from build123d import *

# Parameters (mm, degrees)
CROQUIS1_R              = 60
SALIENTE_EXTRUIR1_DEPTH = 2
CROQUIS2_R              = 60
CROQUIS2_R_2            = 52
SALIENTE_EXTRUIR2_DEPTH = 2.5
CROQUIS3_R              = 1.5875
CORTAR_EXTRUIR1_DEPTH   = 85.97205423
CROQUIS4_R              = 4.75
CORTAR_EXTRUIR2_DEPTH   = 85.97205423
CROQUIS5_R              = 2.1
CORTAR_EXTRUIR3_DEPTH   = 85.97205423


with BuildPart() as part:
    # Croquis1 → Saliente-Extruir1 (new body)
    with BuildSketch(Plane.XY):
        Circle(CROQUIS1_R)
    extrude(amount=SALIENTE_EXTRUIR1_DEPTH)

    # Croquis2 → Saliente-Extruir2 (add)
    with BuildSketch(Plane.XY.offset(2)):
        Circle(CROQUIS2_R)
        Circle(CROQUIS2_R_2, mode=Mode.SUBTRACT)
    extrude(amount=SALIENTE_EXTRUIR2_DEPTH)

    # Croquis3 → Cortar-Extruir1 (cut, through all)
    with BuildSketch(Plane.XY.offset(4.5)):
        with Locations((0, 55.5)):
            Circle(CROQUIS3_R)
        with Locations((48.06440991, -27.75)):
            Circle(CROQUIS3_R)
        with Locations((-48.06440991, -27.75)):
            Circle(CROQUIS3_R)
    extrude(amount=-CORTAR_EXTRUIR1_DEPTH, mode=Mode.SUBTRACT)

    # Croquis4 → Cortar-Extruir2 (cut, through all)
    with BuildSketch(Plane(origin=(0, 0, 0), x_dir=(-1, 0, 0), z_dir=(0, 0, -1))):
        Circle(CROQUIS4_R)
    extrude(amount=-CORTAR_EXTRUIR2_DEPTH, mode=Mode.SUBTRACT)

    # Croquis5 → Cortar-Extruir3 (cut, through all)
    with BuildSketch(Plane(origin=(0, 0, 0), x_dir=(-1, 0, 0), z_dir=(0, 0, -1))):
        with Locations((-17.5, -8)):
            Circle(CROQUIS5_R)
        with Locations((17.5, -8)):
            Circle(CROQUIS5_R)
    extrude(amount=-CORTAR_EXTRUIR3_DEPTH, mode=Mode.SUBTRACT)


solid = part.part
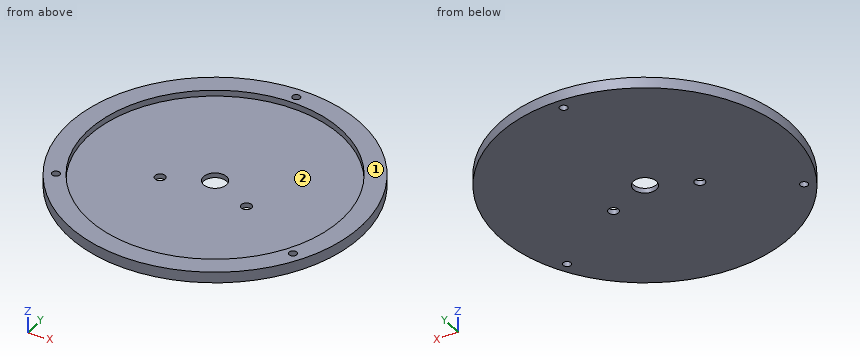
Geometry check sheet. Reference: the model listing, model coordinates, mm. Face numbers are marked on the shaded views. Give positions to 0.01 mm unless a question says otherwise; leave off trailing zeros. Write each loop counter-clockwise with the first axis right and the second up, starting at its lowest first coordinate (ties: lowest second). Pieces come first, ordered by that corner, then holes.
1) Cross-section at A-A (z = 0.8). Count the separate pieces of the cut face and the enclosed holes in it, plus the area to 3 significant figures.
Values follow:
separate pieces: 1
enclosed holes: 6
area: 11,200 mm2
2) Go/stop test with flat-tipped pins: pin 1 Ø5 at (x, y) = (-20, 3) entering from +Z; pin 2 Ø2 at (x, z) = (-24.5, 3.5) entering from -Y; pin 3 Ø3 at (x, y) = (-48.06, -27.75) entering from +Z. Record where each tip stops, or that it passes through.
Values follow:
pin 1: stops at z = 2
pin 2: stops at y = -55.21
pin 3: passes through
3) Release check for a two-part mould opening along X. For the marked faces 1 and 2 record: released by +X, released by -X, zero draft, split by the parting line, or undercut.
Values follow:
face 1: zero draft
face 2: undercut
4) Cross-section at D-D (x = 17.5). Record the boundary of the cut face in (y, z), plus the area to 3 significant figures.
Values follow:
outline: (-57.39, 0) - (-10.1, 0) - (-10.1, 2) - (-48.97, 2) - (-48.97, 4.5) - (-57.39, 4.5) - close; (-5.9, 0) - (57.39, 0) - (57.39, 4.5) - (48.97, 4.5) - (48.97, 2) - (-5.9, 2) - close
area: 263 mm2
5) Cross-section at B-B (y = -8). Record the boundary of the cut face in (x, z).
Values follow:
outline: (-59.46, 0) - (-19.6, 0) - (-19.6, 2) - (-51.38, 2) - (-51.38, 4.5) - (-59.46, 4.5) - close; (-15.4, 0) - (15.4, 0) - (15.4, 2) - (-15.4, 2) - close; (19.6, 0) - (59.46, 0) - (59.46, 4.5) - (51.38, 4.5) - (51.38, 2) - (19.6, 2) - close
6) Cross-section at C-C (x = 0). Record the boundary of the cut face in (y, z), plus the area to 3 significant figures.
Values follow:
outline: (-60, 0) - (-4.75, 0) - (-4.75, 2) - (-52, 2) - (-52, 4.5) - (-60, 4.5) - close; (4.75, 0) - (53.91, 0) - (53.91, 4.5) - (52, 4.5) - (52, 2) - (4.75, 2) - close; (57.09, 0) - (60, 0) - (60, 4.5) - (57.09, 4.5) - close
area: 247 mm2
7) Thickness scan on line 1 (Y direction, x = -47, z = 3.95); line 2 (X direction, y = -27.5, z = 0.3); line 3 (Y direction, x = 0, z = 0.65). Record the ranges inside material, lowest first.
Values follow:
line 1: y = -37.3 to -28.93, -26.57 to -22.25, 22.25 to 37.3
line 2: x = -53.33 to -49.63, -46.5 to 46.5, 49.63 to 53.33
line 3: y = -60 to -4.75, 4.75 to 53.91, 57.09 to 60
